from build123d import *

# Parameters (mm, degrees)
BOSS_EXTRUDE1_DEPTH = 4.7752
FILLET1_R           = 6.35


with BuildPart() as part:
    # Sketch1 → Boss-Extrude1 (new body)
    with BuildSketch(Plane.XY):
        Polygon((170.467651581, -171.615744818), (69.239557334, -171.615744818), (69.239557334, -43.011155522), (56.539557334, -18.443630812), (56.539557334, 31.584255182), (50.8, 31.584255182), (-26.010442666, 31.584255182), (-26.010442666, -19.215744818), (-44.45, -54.886160601), (-44.45, -171.615744818), (-63.5, -171.615744818), (-170.467651581, -171.615744818), (-298.45, 50.056185115), (-298.45, 167.681366782), (-200.025, 205.781366782), (-63.5, 205.781366782), (63.5, 205.781366782), (200.025, 205.781366782), (298.45, 167.681366782), (298.45, 50.056185115), align=None)
    extrude(amount=BOSS_EXTRUDE1_DEPTH)

    # Fillet1
    fillet1_edges = [part.edges().sort_by_distance(p)[0] for p in [
        (69.239557334, -171.615744818, 2.3876),
        (69.239557334, -43.011155522, 2.3876),
        (56.539557334, -18.443630812, 2.3876),
        (56.539557334, 31.584255182, 2.3876),
        (-26.010442666, 31.584255182, 2.3876),
        (-26.010442666, -19.215744818, 2.3876),
        (-44.45, -54.886160601, 2.3876),
        (-44.45, -171.615744818, 2.3876),
    ]]
    fillet(fillet1_edges, radius=FILLET1_R)


solid = part.part
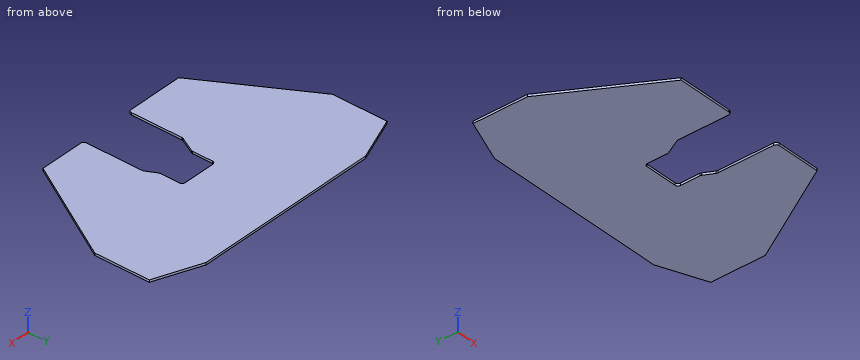
The listing builds one solid part. Answer for the finished solid, in the listing's coordinates (mm). Give positions to 0.01 mm unless a question says otherwise; leave off trailing zeros. Loops run counter-clockwise (first coordinate to the right, second up) from the corner with the lowest first, then second, coordinate; pieces in that order, holes last. Notation, with made-up numbers: M 5,84.5 L 19,84.5 A36 ccw 19,119.5 Z; hole C 25.5,-6 d2. An arc over 180 degrees is marked long. Answer as CSV lines item,"result".
Item 1: The part is cut by section D-D (y = 178.5). Give the vertices of the cut face in (x, z), and give its area (3 significant figures).
Values follow:
outline,"M -270.5,0 L 270.5,0 L 270.5,4.78 L -270.5,4.78 Z"
area,"2,580 mm^2"
Item 2: The part is cut by section B-B (z = 1.9). Give the vertices of the cut face in (x, y) (3 decimals), and give its area (3 significant figures).
Values follow:
outline,"M -298.45,50.056 L -170.468,-171.616 L -50.8,-171.616 A6.35 ccw -44.45,-165.266 L -44.45,-56.43 A6.35 cw -43.741,-53.514 L -26.72,-20.588 A6.35 ccw -26.01,-17.672 L -26.01,25.234 A6.35 cw -19.66,31.584 L 50.19,31.584 A6.35 cw 56.54,25.234 L 56.54,-16.899 A6.35 ccw 57.249,-19.815 L 68.53,-41.639 A6.35 cw 69.24,-44.555 L 69.24,-165.266 A6.35 ccw 75.59,-171.616 L 170.468,-171.616 L 298.45,50.056 L 298.45,167.681 L 200.025,205.781 L -200.025,205.781 L -298.45,167.681 Z"
area,"172,000 mm^2"
Item 3: Straight lines are drawn through the part: line 1 along Y through (x, z) = (10, 1.4); line 2 along X through (y, z) = (17, 2.85) (3 decimals); line 3 along X through (y, z) = (-18, 2). For each, find the intervals that lie inside material, in ascending order. Write a range as [from, to].
Values follow:
line 1,"y = [31.58, 205.78]"
line 2,"x = [-279.365, -26.01], [56.54, 279.365]"
line 3,"x = [-259.16, -26.02], [56.64, 259.16]"
Item 4: The part is cut by section C-C (x = 34.5). Give the vertices of the cut face in (y, z), and give its area (3 significant figures).
Values follow:
outline,"M 31.58,0 L 205.78,0 L 205.78,4.78 L 31.58,4.78 Z"
area,"832 mm^2"
Item 5: The part is cut by section A-A (y = -112). Give the vertices of the cut face in (x, z).
Values follow:
outline,"M -204.89,0 L -44.45,0 L -44.45,4.78 L -204.89,4.78 Z; M 69.24,0 L 204.89,0 L 204.89,4.78 L 69.24,4.78 Z"
Item 6: Given pin 1 Ø2 at (x, z) = (16, 4) entering from -Y; pin 2 Ø2 at (y, z) = (42, 4) entering from -X; pin 3 Ø2.5 at (y, z) = (-5, 2) entering from +X (3 decimals), each flat-ended and moving along its own axis, determine where each tip first touches the part or whether it passes through.
Values follow:
pin 1,"stops at y = 31.58"
pin 2,"stops at x = -294.38"
pin 3,"stops at x = 267.385"
